The drawing under review shows one solid part. Ordinate dimensions are in mm from its lowest x, y, z. Give positions to 0.01 mm unless a question says otherwise; leave off trailing zeros. Loops run counter-clockwise (first coordinate to the right, second up) from the corner with the lowest first, then second, coordinate; pieces in that order, holes last. Notation, with made-up numbers: (-6, 12) - (17, 12) arc R15 cw to (17, 40) - close; hole circle Ø7 at (12.5, -9). An arc over 180 degrees is marked (long way). Answer as CSV lines item,"result".
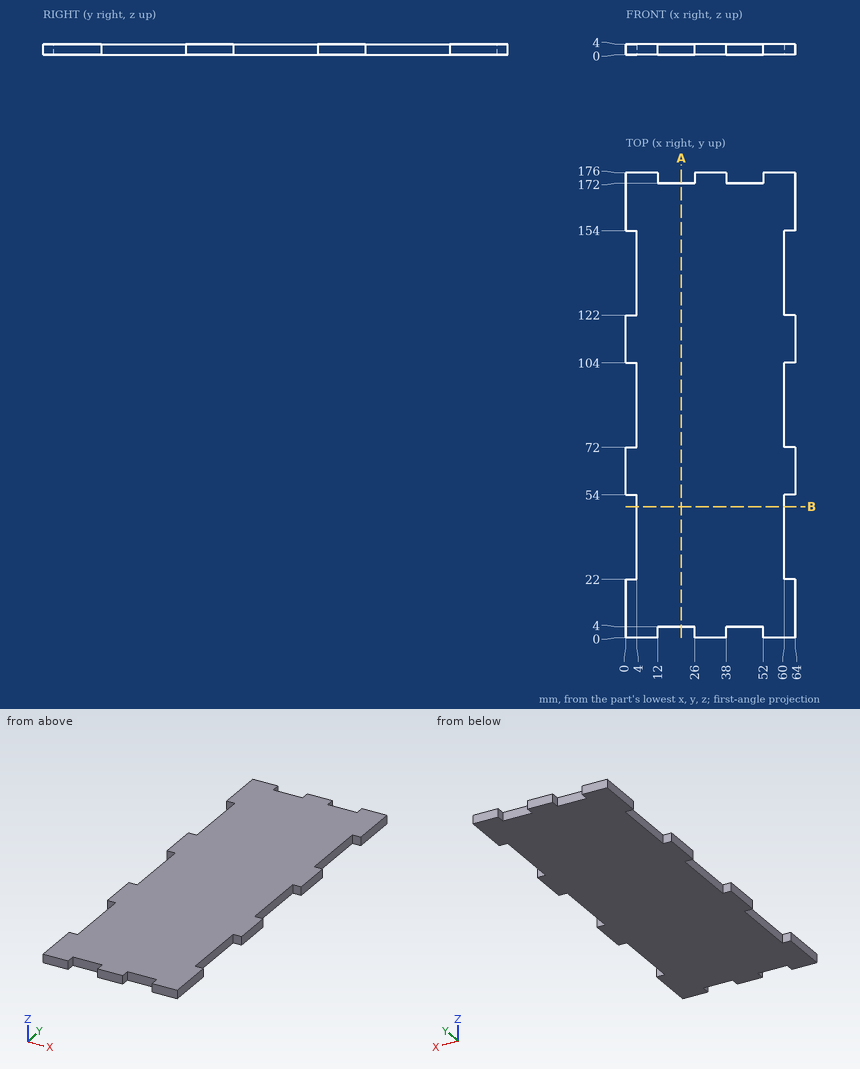
1) Wall thickness on line 1 (X direction, y = 47.5, z = 1.1); line 2 (Y direction, x = 46.5, z = 1.25): over which ranges is each line inside the solid? List them lowest first. Write a range as from..to.
From the geometry:
line 1,"x = 4..60"
line 2,"y = 4..172"
2) Consider section B-B on y = 49.5. Write out the cut boundary in (x, z).
From the geometry:
outline,"(4, 0) - (60, 0) - (60, 4) - (4, 4) - close"
3) Consider section A-A on x = 21. Write out the cut boundary in (y, z).
From the geometry:
outline,"(4, 0) - (172, 0) - (172, 4) - (4, 4) - close"
4) Insertion check: P1, Ø1.2, axis at y = 82, z = 3, coming from the +X side; P2, Ø1.5, axis at y = 86, z = 3.5, coming from the -X side; P3, Ø1.5, axis at x = 19.5, z = 1.5, coming from the -Y side. Each pin has a flat end and moves straight along its axis. Give the tip position at first contact, or say it passes through.
From the geometry:
P1,"stops at x = 60"
P2,"stops at x = 4"
P3,"stops at y = 4"
